from build123d import *

# Parameters (mm, degrees)
BOSS_EXTRUDE1_DEPTH = 10
SKETCH2_R           = 2.625
CUT_EXTRUDE1_DEPTH  = 69.02664919
SKETCH3_R           = 2.625
CUT_EXTRUDE2_DEPTH  = 108.332520819
CUT_EXTRUDE3_DEPTH  = 11
FILLET1_R           = 10
CHAMFER1_SIZE       = 8


with BuildPart() as part:
    # Sketch1 → Boss-Extrude1 (new, symmetric)
    with BuildSketch(Plane(origin=(0, 0, 0), x_dir=(1, 0, 0), z_dir=(0, 1, 0))):
        with BuildLine():
            Line((-37.693666577, 6.5), (-50.25, 6.5))
            Line((-50.25, 6.5), (-50.25, 3))
            Line((-50.25, 3), (-36.627346341, 3))
            ThreePointArc((-36.627346341, 3), (3.731967617, 36.560018021), (36.478063401, -4.462442214))
            Line((36.478063401, -4.462442214), (38.147922337, -2.792583278))
            ThreePointArc((38.147922337, -2.792583278), (4.651839751, 37.966075474), (-37.693666577, 6.5))
        make_face()
        with BuildLine():
            Line((48.754524055, -13.399184996), (38.147922337, -2.792583278))
            ThreePointArc((38.147922337, -2.792583278), (27.04683438, -27.04683438), (2.792583278, -38.147922337))
            Line((2.792583278, -38.147922337), (13.399184996, -48.754524055))
            Line((13.399184996, -48.754524055), (48.754524055, -13.399184996))
        make_face()
        with BuildLine():
            ThreePointArc((-37.693666577, -6.5), (-23.55672199, -30.135416856), (2.792583278, -38.147922337))
            Line((2.792583278, -38.147922337), (4.462442214, -36.478063401))
            ThreePointArc((4.462442214, -36.478063401), (-23.212937054, -28.490736272), (-36.627346341, -3))
            Line((-36.627346341, -3), (-50.25, -3))
            Line((-50.25, -3), (-50.25, -6.5))
            Line((-50.25, -6.5), (-37.693666577, -6.5))
        make_face()
        with BuildLine():
            ThreePointArc((2.792583278, -38.147922337), (27.04683438, -27.04683438), (38.147922337, -2.792583278))
            Line((38.147922337, -2.792583278), (36.478063401, -4.462442214))
            ThreePointArc((36.478063401, -4.462442214), (25.986174209, -25.986174209), (4.462442214, -36.478063401))
            Line((4.462442214, -36.478063401), (2.792583278, -38.147922337))
        make_face()
    extrude(amount=BOSS_EXTRUDE1_DEPTH, both=True)

    # Sketch2 → Cut-Extrude1 (cut, through all)
    with BuildSketch(Plane.XY.offset(6.5)):
        with Locations((-44.008194531, 0)):
            Circle(SKETCH2_R)
    extrude(amount=-CUT_EXTRUDE1_DEPTH, mode=Mode.SUBTRACT)

    # Sketch3 → Cut-Extrude2 (cut, through all)
    with BuildSketch(Plane(origin=(31.076854525, 0, 31.076854525), x_dir=(0.7071067811865457, 0, -0.7071067811865496), z_dir=(0.7071067811865496, 0, 0.7071067811865457))):
        Circle(SKETCH3_R)
        with Locations((-12.5, 0)):
            Circle(SKETCH3_R)
        with Locations((12.5, 0)):
            Circle(SKETCH3_R)
    extrude(amount=-CUT_EXTRUDE2_DEPTH, mode=Mode.SUBTRACT)

    # Sketch6 → Cut-Extrude3 (cut)
    with BuildSketch(Plane(origin=(20.470252807, 0, 20.470252807), x_dir=(0.7071067811865457, 0, -0.7071067811865495), z_dir=(0.7071067811865495, 0, 0.7071067811865457))):
        with BuildLine():
            Line((12.5, -5.5), (-12.5, -5.5))
            ThreePointArc((-12.5, -5.5), (-18, 0), (-12.5, 5.5))
            Line((-12.5, 5.5), (12.5, 5.5))
            ThreePointArc((12.5, 5.5), (18, 0), (12.5, -5.5))
        make_face()
    extrude(amount=CUT_EXTRUDE3_DEPTH, mode=Mode.SUBTRACT)

    # Fillet1
    fillet1_edges = [part.edges().sort_by_distance(p)[0] for p in [
        (-50.25, -10, 4.75),
        (-50.25, 10, 4.75),
        (-50.25, -10, -4.75),
        (-50.25, 10, -4.75),
    ]]
    fillet(fillet1_edges, radius=FILLET1_R - 0.0001)  # a hair under: the kernel refuses the full size

    # Chamfer1
    chamfer1_edges = [part.edges().sort_by_distance(p)[0] for p in [
        (48.754524055, 0, 13.399184996),
        (13.399184996, 0, 48.754524055),
    ]]
    chamfer(chamfer1_edges, length=CHAMFER1_SIZE)


solid = part.part
The model under review builds one solid part; all positions refer to its coordinate system, in mm. A direction names the side the tool comes from. Coordinates: 2 decimals unless noted, no trailing zeros. Write each loop counter-clockwise with the first axis right and the second up, starting at its lowest first coordinate (ties: lowest second). Pieces come first, ordered by that corner, then holes. Notation, with made-up numbers: (-28, -8) - (-22, -8) arc R13 ccw to (-22, 3) - close; hole circle Ø7 at (-23.5, -16). An arc over 180 degrees is marked (long way). Answer as a JSON object with one key per item and string values. Group by question number.
1. Add section C-C (y = 3.75). Give the boundary of the cut face in (x, z).
2. Machinability: for faces 1 (the face through (13.307, -0.121, 38.761)), 2 (the face through (-41, 0, -6.5)), 3 (the face through (-41.504, 0.788, 4.774)), which of the approach directions +Z, -Z, +X, -X, +Y, -Y give a long, thin tool a straight path to every point of the face, cutting with its end or side? Answer none if there is none.
3. Add section A-A (x = 0). Give the boundary of the cut face in (y, z).
4. Add section D-D (z = 0). Give the boundary of the cut face in (x, y).
5. Add section B-B (z = -9.5). Give the boundary of the cut face in (x, y), plus the area to 3 significant figures.
6. Mouldability with a two-part tool opening along Z and no side actions: class faces 4 (the face through (-41, 0, 6.5)), 5 (the face through (-47.24, -7.15, 4.77)), 6 (the face through (40.236, -1.005, 19.129)), 7 (the face through (27, 5.5, 27)) as pulls with the +Z half, pulls with the -Z half, needs draft (parallel to the pull), parting line crosses it, or undercut.
7. To check wall thickness, follow probe 1 along Z at (x, y) = (0, -4.75); probe 2 along Z at (x, y) = (26.5, 5); probe 3 along X at (y, z) = (-6.75, 26). State the ranges of each line that lie inside material, in increasing order.
8. Clearance check with flat-ended pins moving along their axes: pin 1 Ø3 at (x, y) = (-44.01, 0) entering from +Z; pin 2 Ø1.5 at (x, y) = (15, 4) entering from -Z; pin 3 Ø23.5 at (x, z) = (25.5, 21.5) entering from +Y; pin 4 Ø6 at (x, y) = (-9.5, 1) entering from +Z. State where each tip first meets the part, or that it passes through.
Findings:
{
 "1": {"outline": "(-49.52, -6.5) - (-37.69, -6.5) arc R38.25 ccw to (38.15, 2.79) - (43.1, 7.74) - (43.1, 19.06) - (19.06, 43.1) - (7.74, 43.1) - (2.79, 38.15) arc R38.25 ccw to (-37.69, 6.5) - (-49.52, 6.5) - (-49.52, 3) - (-36.63, 3) arc R36.75 cw to (11.53, 34.9) - (16.56, 39.93) - (39.93, 16.56) - (34.9, 11.53) arc R36.75 cw (long way) to (-36.63, -3) - (-49.52, -3) - close"},
 "2": {"face 1": "none", "face 2": "-Z, -X, +Y, -Y", "face 3": "+Z, -Z"},
 "3": {"outline": "(-10, -38.25) - (10, -38.25) - (10, -36.75) - (-10, -36.75) - close; (-10, 36.75) - (10, 36.75) - (10, 38.25) - (-10, 38.25) - close"},
 "4": {"outline": "(36.75, -10) - (38.25, -10) - (38.25, 10) - (36.75, 10) - close"},
 "5": {"outline": "(-37.05, -10) - (-35.5, -10) - (-35.5, 10) - (-37.05, 10) - close; (35.5, -10) - (37.05, -10) - (37.05, 10) - (35.5, 10) - close", "area": "62.0 mm²"},
 "6": {"face 4": "pulls with the +Z half", "face 5": "needs draft", "face 6": "undercut", "face 7": "undercut"},
 "7": {"probe 1": "-38.25 to -36.75, 36.75 to 38.25", "probe 2": "-27.58 to -25.46, 30 to 35.65", "probe 3": "-28.05 to -25.97, 25.97 to 36.15"},
 "8": {"pin 1": "through", "pin 2": "z = -35.5", "pin 3": "y = 10", "pin 4": "z = 37.69"}
}
